Geometry check sheet. Reference: the model listing, model coordinates, mm. Face numbers are marked on the shaded views. A direction names the side the tool comes from. Round coordinates to 2 decimals unless told otherwise and drop trailing zeros. Order: outer loops, then holes, each group sorted by start corner. A loop starts at its lowest first (then second) coordinate and runs counter-clockwise, first axis right, second up. Notation, with made-up numbers: (20.25, 10.25) - (74.25, 10.25) arc R14 cw to (74.25, 24.25) - close; hole circle Ø11 at (71.25, 77.25). An arc over 180 degrees is marked (long way). Use a Markdown table: item, result. Add a question column.
(1) Access from +Z, -Z, +X, -X, +Y, -Y to the whole of each face (thin tool, end or side, straight path). Record for the marked faces 4, 5, 6 and 7.
(2) Mould release check, pull along Z, two halves, no side actions. Record for the marked faces 1, 2 and 3: released by +Z, released by -Z, zero draft, split by the parting line, or undercut.
(3) Section check A-A on y = 0. Record the boundary of the cut face in (x, z).
(4) Section check D-D on x = -36.5. Record the boundary of the cut face in (y, z), then the cut area to 3 significant figures.
(5) Gauge pin test, flat ends, axial feed: P1, Ø2, axis at x = -42, z = 6, coming from the -Y side; P2, Ø6, axis at x = -50.5, z = -2, coming from the +Y side; P3, Ø1.2, axis at y = -19.5, z = -4.5, coming from the -X side. Record the tip position at first contact, or that the pin passes through.
(6) Section check B-B on x = 11. Record the boundary of the cut face in (y, z), then the cut area to 3 significant figures.
(7) Thickness scan on line 1 along X through (y, z) = (-20, -19.5); line 2 along Y through (x, z) = (-23, -24); line 3 along Y through (x, z) = (-42.75, 0). Record the ranges inside material, lowest first. Write a range as [from, to].
(8) Section check C-C on z = 0. Record the boundary of the cut face in (x, y).
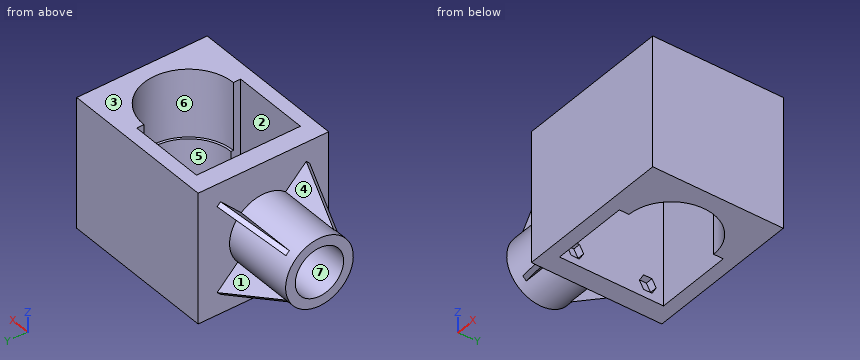
```python
from build123d import *

# Parameters (mm, degrees)
BOSS_EXTRUDE1_DEPTH = 27
SKETCH10_R          = 14
BOSS_EXTRUDE5_DEPTH = 30
SKETCH2_R           = 10
CUT_EXTRUDE7_DEPTH  = 30
BOSS_EXTRUDE9_DEPTH = 1
CIRPATTERN1_COUNT   = 2
CIRPATTERN1_ANGLE   = 90
CUT_EXTRUDE8_DEPTH  = 28
CUT_EXTRUDE9_DEPTH  = 26
CUT_EXTRUDE10_DEPTH = 87.897928629
CUT_EXTRUDE11_DEPTH = 3


with BuildPart() as part:
    # Sketch1 → Boss-Extrude1 (new, symmetric)
    with BuildSketch(Plane(origin=(0, 0, 0), x_dir=(1, 0, 0), z_dir=(0, 1, 0))):
        Polygon((32.5, -27), (32.5, 27), (-32.5, 27), (-32.5, -27), (-20, -27), align=None)
    extrude(amount=BOSS_EXTRUDE1_DEPTH, both=True)

    # Sketch10 → Boss-Extrude5 (add)
    with BuildSketch(Plane(origin=(-32.5, 0, 0), x_dir=(0, 0, -1), z_dir=(1, 0, 0))):
        Circle(SKETCH10_R)
    extrude(amount=-BOSS_EXTRUDE5_DEPTH)

    # Sketch2 → Cut-Extrude7 (cut)
    with BuildSketch(Plane.ZY.offset(32.5)):
        with Locations(Location((0, 0, 0), (0, 0, 180))):
            Circle(SKETCH2_R)
    extrude(amount=CUT_EXTRUDE7_DEPTH, mode=Mode.SUBTRACT)

    # Sketch16 → Boss-Extrude9 (add, symmetric)
    with BuildSketch(Plane(origin=(0, 0, 0), x_dir=(-1, 0, 0), z_dir=(0, 0.7071067811865475, -0.7071067811865477))):
        Polygon((62.5, -12), (30, -12), (32.5, -26.063797676), align=None)
        Polygon((30, 12), (32.5, 26.063797676), (62.5, 12), align=None)
    boss_extrude9 = extrude(amount=BOSS_EXTRUDE9_DEPTH, both=True)

    # CirPattern1: Boss-Extrude9 ×2 about axis
    cirpattern1_axis = Axis((0, 0, 0), (1, 0, 0))
    for i in range(1, CIRPATTERN1_COUNT):
        add(boss_extrude9.rotate(cirpattern1_axis, i * CIRPATTERN1_ANGLE / (CIRPATTERN1_COUNT - 1)))

    # Sketch18 → Cut-Extrude8 (cut)
    with BuildSketch(Plane.XY.offset(27)):
        with BuildLine():
            Line((7.5, -18.5), (-2.5, -18.5))
            ThreePointArc((-2.5, -18.5), (-21, 0), (-2.5, 18.5))
            Line((-2.5, 18.5), (7.5, 18.5))
            ThreePointArc((7.5, 18.5), (26, 0), (7.5, -18.5))
        make_face()
    extrude(amount=-CUT_EXTRUDE8_DEPTH, mode=Mode.SUBTRACT)

    # Sketch19 → Cut-Extrude9 (cut)
    with BuildSketch(Plane(origin=(0, 0, -27), x_dir=(-1, 0, 0), z_dir=(0, 0, -1))):
        with BuildLine():
            Line((2.5, -17.5), (-7.5, -17.5))
            ThreePointArc((-7.5, -17.5), (-25, 0), (-7.5, 17.5))
            Line((-7.5, 17.5), (2.5, 17.5))
            ThreePointArc((2.5, 17.5), (20, 0), (2.5, -17.5))
        make_face()
    extrude(amount=-CUT_EXTRUDE9_DEPTH, mode=Mode.SUBTRACT)

    # Sketch20 → Cut-Extrude10 (cut, through all)
    with BuildSketch(Plane.XY.offset(27)):
        Polygon((-24.5, 21.5), (-24.5, -21.5), (7.5, -21.5), (7.5, -18.5), (7.5, 18.5), (7.5, 21.5), align=None)
    extrude(amount=-CUT_EXTRUDE10_DEPTH, mode=Mode.SUBTRACT)

    # Sketch22 → Cut-Extrude11 (cut)
    with BuildSketch(Plane(origin=(-24.5, 0, 0), x_dir=(0, 0, -1), z_dir=(1, 0, 0))):
        Polygon((18, -16.732050808), (21, -18.464101615), (24, -16.732050808), (24, -13.267949192), (21, -11.535898385), (18, -13.267949192), align=None)
        Polygon((-24, -16.732050808), (-21, -18.464101615), (-18, -16.732050808), (-18, -13.267949192), (-21, -11.535898385), (-24, -13.267949192), align=None)
        Polygon((-24.464101615, 15), (-22.732050808, 12), (-19.267949192, 12), (-17.535898385, 15), (-19.267949192, 18), (-22.732050808, 18), align=None)
        Polygon((18, 16.732050808), (18, 13.267949192), (21, 11.535898385), (24, 13.267949192), (24, 16.732050808), (21, 18.464101615), align=None)
    extrude(amount=-CUT_EXTRUDE11_DEPTH, mode=Mode.SUBTRACT)


solid = part.part
```
Check sheet entries:
| question | item | result |
|---|---|---|
| 1 | face 4 | +Z, -X |
| 1 | face 5 | +Z, -Z |
| 1 | face 6 | +Z |
| 1 | face 7 | -X |
| 2 | face 1 | undercut |
| 2 | face 2 | zero draft |
| 2 | face 3 | released by +Z |
| 3 | outline | (-62.5, -14) - (-32.5, -14) - (-32.5, -27) - (-24.5, -27) - (-24.5, 27) - (-32.5, 27) - (-32.5, 14) - (-62.5, 14) - (-62.5, 10) - (-32.5, 10) - (-32.5, -10) - (-62.5, -10) - close; (25, -27) - (32.5, -27) - (32.5, 27) - (26, 27) - (26, -1) - (25, -1) - close |
| 4 | outline | (-17.81, -16.4) - (-16.4, -17.81) - (-9.17, -10.58) arc R14 ccw to (9.17, -10.58) - (16.4, -17.81) - (17.81, -16.4) - (10.58, -9.17) arc R14 ccw to (10.58, 9.17) - (17.81, 16.4) - (16.4, 17.81) - (9.17, 10.58) arc R14 ccw to (-9.17, 10.58) - (-16.4, 17.81) - (-17.81, 16.4) - (-10.58, 9.17) arc R14 ccw to (-10.58, -9.17) - close; hole circle Ø20 at (0, 0) |
| 4 | area | 383 mm2 |
| 5 | P1 | stops at y = -13.08 |
| 5 | P2 | stops at y = 14 |
| 5 | P3 | stops at x = -32.5 |
| 6 | outline | (-27, -27) - (-17.15, -27) - (-17.15, -1) - (-18.17, -1) - (-18.17, 27) - (-27, 27) - close; (17.15, -27) - (27, -27) - (27, 27) - (18.17, 27) - (18.17, -1) - (17.15, -1) - close |
| 6 | area | 1,010 mm2 |
| 7 | line 1 | x = [-32.5, -24.5], [7.5, 32.5] |
| 7 | line 2 | y = [-27, -21.5], [21.5, 27] |
| 7 | line 3 | y = [-14, -10], [10, 14] |
| 8 | outline | (-62.5, -14) - (-32.5, -14) - (-32.5, -27) - (32.5, -27) - (32.5, 27) - (-32.5, 27) - (-32.5, 14) - (-62.5, 14) - (-62.5, 10) - (-32.5, 10) - (-32.5, -10) - (-62.5, -10) - close; hole (-24.5, -21.5) - (7.5, -21.5) - (7.5, -18.5) arc R18.5 ccw to (7.5, 18.5) - (7.5, 21.5) - (-24.5, 21.5) - close |
